Input: part model. Units: mm. Frame: model coordinates. A direction names the side the tool comes from. Give positions to 0.01 mm unless a question says otherwise; leave off trailing zeros. Loops run counter-clockwise (first coordinate to the right, second up) from the corner with the lowest first, then second, coordinate; pieces in that order, holes last.
from build123d import *

# Parameters (mm, degrees)
ESBO_O1_W                = 100
ESBO_O1_H                = 100
EXTRUS_O1_DEPTH          = 3
EXTRUS_O2_DEPTH          = 9
ESBO_O3_W                = 12.7
ESBO_O3_H                = 41
EXTRUS_O3_DEPTH          = 9
FILETE2_R                = 3
ESBO_O6_W                = 3
ESBO_O6_H                = 10
EXTRUS_O4_DEPTH          = 3
ESBO_O7_W                = 3
ESBO_O7_H                = 10
EXTRUS_O5_DEPTH          = 17
EXTRUS_O6_DEPTH          = 8
FILETE3_R                = 3
FILETE2_OF_ESPELHAR4_R   = 3
FILETE3_OF_ESPELHAR4_R   = 3
EXTRUS_O17_DEPTH         = 10
EXTRUS_O30_DEPTH         = 10
ESBO_O22_W               = 100
ESBO_O22_H               = 3
EXTRUS_O33_DEPTH         = 53
ESBO_O23_W               = 100
ESBO_O23_H               = 53
EXTRUS_O35_DEPTH         = 10
ESBO_O24_W               = 50
ESBO_O24_H               = 10
EXTRUS_O36_DEPTH         = 148.030904796
RESSALTO_EXTRUS_O1_DEPTH = 55


with BuildPart() as part:
    # Esboço1 → Extrusão1 (new body)
    with BuildSketch(Plane(origin=(0, 0, 0), x_dir=(1, 0, 0), z_dir=(0, 1, 0))):
        Rectangle(ESBO_O1_W, ESBO_O1_H)
    extrus_o1 = extrude(amount=EXTRUS_O1_DEPTH)

    # Esboço2 → Extrusão2 (add)
    with BuildSketch(Plane(origin=(0, 3, 0), x_dir=(1, 0, 0), z_dir=(0, 1, 0))):
        Polygon((-50, -3), (-31.3, -3), (-31.3, -50), (-50, -50), (-50, -23), (-53, -23), (-53, -13), (-50, -13), align=None)
    extrus_o2 = extrude(amount=EXTRUS_O2_DEPTH)

    # Esboço3 → Extrusão3 (cut)
    with BuildSketch(Plane(origin=(0, 12, 0), x_dir=(-1, 0, 0), z_dir=(0, 1, 0))):
        with Locations((40.65, 26.5)):
            Rectangle(ESBO_O3_W, ESBO_O3_H)
    extrus_o3 = extrude(amount=-EXTRUS_O3_DEPTH, mode=Mode.SUBTRACT)

    # Filete2
    filete2_edges = [part.edges().sort_by_distance(p)[0] for p in [
        (-50, 7.5, 3),
        (-31.3, 7.5, 3),
    ]]
    fillet(filete2_edges, radius=FILETE2_R)

    # Esboço6 → Extrusão4 (add)
    with BuildSketch(Plane.XZ.offset(-3)):
        with Locations((-51.5, 18)):
            Rectangle(ESBO_O6_W, ESBO_O6_H)
    extrus_o4 = extrude(amount=EXTRUS_O4_DEPTH)

    # Esboço7 → Extrusão5 (add)
    with BuildSketch(Plane(origin=(0, 3, 0), x_dir=(1, 0, 0), z_dir=(0, 1, 0))):
        with Locations((-29.8, -18)):
            Rectangle(ESBO_O7_W, ESBO_O7_H)
    extrus_o5 = extrude(amount=EXTRUS_O5_DEPTH)

    # Esboço8 → Extrusão6 (add)
    with BuildSketch(Plane(origin=(0, 12, 0), x_dir=(1, 0, 0), z_dir=(0, 1, 0))):
        Polygon((-53.00042216, -13), (-50.053356487, -13), (-50, -23), (-53, -23), align=None)
    extrus_o6 = extrude(amount=EXTRUS_O6_DEPTH)

    # Filete3
    filete3_edges = [part.edges().sort_by_distance(p)[0] for p in [
        (-51.5, 20, 23),
        (-51.526889323, 20, 13),
        (-29.8, 20, 23),
        (-29.8, 20, 13),
    ]]
    fillet(filete3_edges, radius=FILETE3_R)

    # Espelhar4: Extrusão1, Extrusão2, Extrusão3, Extrusão4, Extrusão5, Extrusão6 across plane
    add(extrus_o1.mirror(Plane(origin=(0, 0, 0), x_dir=(0, 0, 1), z_dir=(1, 0, 0))))
    add(extrus_o2.mirror(Plane(origin=(0, 0, 0), x_dir=(0, 0, 1), z_dir=(1, 0, 0))))
    add(extrus_o3.mirror(Plane(origin=(0, 0, 0), x_dir=(0, 0, 1), z_dir=(1, 0, 0))), mode=Mode.SUBTRACT)
    add(extrus_o4.mirror(Plane(origin=(0, 0, 0), x_dir=(0, 0, 1), z_dir=(1, 0, 0))))
    add(extrus_o5.mirror(Plane(origin=(0, 0, 0), x_dir=(0, 0, 1), z_dir=(1, 0, 0))))
    add(extrus_o6.mirror(Plane(origin=(0, 0, 0), x_dir=(0, 0, 1), z_dir=(1, 0, 0))))

    # Filete2 of Espelhar4
    filete2_of_espelhar4_edges = [part.edges().sort_by_distance(p)[0] for p in [
        (50, 7.5, 3),
        (31.3, 7.5, 3),
    ]]
    fillet(filete2_of_espelhar4_edges, radius=FILETE2_OF_ESPELHAR4_R)

    # Filete3 of Espelhar4
    filete3_of_espelhar4_edges = [part.edges().sort_by_distance(p)[0] for p in [
        (51.5, 20, 23),
        (51.526889323, 20, 13),
        (29.8, 20, 23),
        (29.8, 20, 13),
    ]]
    fillet(filete3_of_espelhar4_edges, radius=FILETE3_OF_ESPELHAR4_R)

    # Esboço9 → Extrusão17 (cut)
    with BuildSketch(Plane(origin=(-28.3, 0, 0), x_dir=(0, 0, -1), z_dir=(1, 0, 0))):
        with BuildLine():
            ThreePointArc((-18, 17.5), (-19.060660172, 17.060660172), (-19.5, 16))
            Line((-19.5, 16), (-19.5, 13.5))
            ThreePointArc((-19.5, 13.5), (-19.060660172, 12.439339828), (-18, 12))
            ThreePointArc((-18, 12), (-16.939339828, 12.439339828), (-16.5, 13.5))
            Line((-16.5, 13.5), (-16.5, 16))
            ThreePointArc((-16.5, 16), (-16.939339828, 17.060660172), (-18, 17.5))
        make_face()
    extrus_o17 = extrude(amount=-EXTRUS_O17_DEPTH, mode=Mode.SUBTRACT)

    # Esboço15 → Extrusão30 (cut)
    with BuildSketch(Plane(origin=(-50.121293009, 0, 0.267429611), x_dir=(-0.005335572730928429, 0, -0.9999857657305093), z_dir=(0.9999857657305093, 0, -0.005335572730928429))):
        with BuildLine():
            Line((-19.232893975, 16.01), (-19.232893975, 13.51))
            ThreePointArc((-19.232893975, 13.51), (-17.732893975, 12.01), (-16.232893975, 13.51))
            Line((-16.232893975, 13.51), (-16.232893975, 16.01))
            ThreePointArc((-16.232893975, 16.01), (-17.732893975, 17.51), (-19.232893975, 16.01))
        make_face()
    extrus_o30 = extrude(amount=-EXTRUS_O30_DEPTH, mode=Mode.SUBTRACT)

    # Espelhar14: Extrusão17, Extrusão30 across plane
    add(extrus_o17.mirror(Plane(origin=(0, 0, 0), x_dir=(0, 0, 1), z_dir=(1, 0, 0))), mode=Mode.SUBTRACT)
    add(extrus_o30.mirror(Plane(origin=(0, 0, 0), x_dir=(0, 0, 1), z_dir=(1, 0, 0))), mode=Mode.SUBTRACT)

    # Esboço22 → Extrusão33 (add)
    with BuildSketch(Plane(origin=(0, 0, -50), x_dir=(-1, 0, 0), z_dir=(0, 0, -1))):
        with Locations((0, 1.5)):
            Rectangle(ESBO_O22_W, ESBO_O22_H)
    extrude(amount=EXTRUS_O33_DEPTH)

    # Esboço23 → Extrusão35 (add)
    with BuildSketch(Plane(origin=(0, 3, 0), x_dir=(1, 0, 0), z_dir=(0, 1, 0))):
        with Locations((0, 76.5)):
            Rectangle(ESBO_O23_W, ESBO_O23_H)
    extrude(amount=EXTRUS_O35_DEPTH)

    # Esboço24 → Extrusão36 (cut, through all)
    with BuildSketch(Plane(origin=(50, 0, 0), x_dir=(0, 0, -1), z_dir=(1, 0, 0))):
        with Locations((78, 5)):
            Rectangle(ESBO_O24_W, ESBO_O24_H)
    extrude(amount=-EXTRUS_O36_DEPTH, mode=Mode.SUBTRACT)

    # Esboço26 → Ressalto-extrusão1 (add)
    with BuildSketch(Plane.XY.offset(50)):
        Polygon((31.3, 3), (-31.3, 3), (-50, 3), (-50, 0), (50, 0), (50, 3), align=None)
    extrude(amount=RESSALTO_EXTRUS_O1_DEPTH)


solid = part.part
(1) Cut plane C-C (y = 7). Count the separate pieces of the cut face and the enclosed holes in it, and give its area (3 significant figures).
Values follow:
separate pieces: 3
enclosed holes: 2
area: 1,130 mm2
(2) Cut plane A-A (z = 39.5). Return the cut outline in (x, y), and give its area (3 significant figures).
Values follow:
outline: (-50, 0) - (50, 0) - (50, 12) - (47, 12) - (47, 3) - (34.3, 3) - (34.3, 12) - (31.3, 12) - (31.3, 3) - (-31.3, 3) - (-31.3, 12) - (-34.3, 12) - (-34.3, 3) - (-47, 3) - (-47, 12) - (-50, 12) - close
area: 408 mm2
(3) Cut plane B-B (x = 43). Return the cut outline in (y, z).
Values follow:
outline: (0, -53) - (10, -53) - (10, -103) - (13, -103) - (13, -50) - (3, -50) - (3, 3) - (12, 3) - (12, 6) - (3, 6) - (3, 47) - (12, 47) - (12, 50) - (3, 50) - (3, 105) - (0, 105) - close
(4) Reachability of faces 4 (the flat face through (41, 7, 3)), 5 (the flat face through (-50, 5, 45)), 6 (the flat face through (50, 2.6, -31.8)), 7 (the flat face through (28.3, 11, 18)), 8 (the flat face through (-47, 8, 26)) from +Z, -Z, +X, -X, +Y, -Y: full face, straight path, thin tool, end or side. Return the list, or none.
Values follow:
face 4: +X, -X, +Y
face 5: +Z, -X, +Y, -Y
face 6: -Z, +X, +Y, -Y
face 7: +Z, +Y
face 8: +Y
(5) Ray query, probe 1 along X at (y, z) = (10.5, 40.5); probe 2 along X at (y, z) = (13, 22); probe 3 along Z at (x, y) = (46.5, 9). Return the intervals inside material, ascending.
Values follow:
probe 1: x = -50 to -47, -34.3 to -31.3, 31.3 to 34.3, 47 to 50
probe 2: x = -53 to -50.01, -31.3 to -28.3, 28.3 to 31.3, 50.01 to 53
probe 3: z = -53 to -50, 3 to 6, 47 to 50
(6) Mould query, pull axis Z, two halves, no side actions, for faces 1 (the flat face through (41, 3, 27)), 2 (the flat face through (53, 6, 18)), 3 (the flat face through (1, 5, -53)). Classes: +Z half, -Z half, draft (parallel to the pull), parting line (faces both ways), or undercut.
Values follow:
face 1: undercut
face 2: draft
face 3: -Z half
(7) Pin query (flat end, axial travel): pin 1 Ø8 at (x, y) = (23.5, 10) entering from +Z; pin 2 Ø12 at (y, z) = (7, -6) entering from -X; pin 3 Ø4.5 at (x, y) = (40.5, 7) entering from +Z. Return the tip coordinate at first contact, or that it passes through.
Values follow:
pin 1: stops at z = -50
pin 2: stops at x = -50
pin 3: stops at z = 50
(8) Cut plane D-D (x = -7). Return the cut outline in (y, z).
Values follow:
outline: (0, -53) - (10, -53) - (10, -103) - (13, -103) - (13, -50) - (3, -50) - (3, 105) - (0, 105) - close
